```python
from build123d import *

# Parameters (mm, degrees)
F0_R     = 21.6611468636
F1_DEPTH = 12
F5_DEPTH = 15
F8_DEPTH = 32.9
F9_DEPTH = 5


with BuildPart() as f1:
    # F0 (on Top) → F1 (new body)
    with BuildSketch(Plane.XY):
        Polygon((-20.2222224325, 30.916666612), (-27.0277783275, 30.916666612), (-27.0277783275, 0), (-27.0277783275, -30.916666612), (-20.2222224325, -30.916666612), (-10.3055555373, -25.6666671485), (0, -25.6666671485), (10.3055555373, -25.6666671485), (20.2222224325, -30.916666612), (27.0277783275, -30.916666612), (27.0277783275, 0), (27.0277783275, 30.916666612), (20.2222224325, 30.916666612), (10.3055555373, 25.6666671485), (0, 25.6666671485), (-10.3055555373, 25.6666671485), align=None)
        Circle(F0_R, mode=Mode.SUBTRACT)
        Circle(F0_R)
    extrude(amount=-F1_DEPTH)

    # F4 (on plane+point) → F5 (join)
    with BuildSketch(Plane(origin=(-27.0277783275, 0, 0), x_dir=(0, -1, 0), z_dir=(-1, 0, 0))):
        with BuildLine():
            ThreePointArc((-37.3333357275, 1.750000054), (-45.7916693995, -6.708333618), (-37.3333357275, -15.16666729))
            Line((-37.3333357275, -15.16666729), (37.138890475, -15.16666729))
            ThreePointArc((37.138890475, -15.16666729), (45.5972241471, -6.708333618), (37.138890475, 1.750000054))
            Line((37.138890475, 1.750000054), (-37.3333357275, 1.750000054))
        make_face()
    extrude(amount=F5_DEPTH)

    # F6: F1 across plane


with BuildPart() as f1_1:
    add(f1.part)
    add(f1.part.mirror(Plane.YZ))

    # F7 (on Front) → F8 (cut, symmetric)
    with BuildSketch(Plane.XZ):
        Polygon((11.4722223952, -5.0555560738), (0, -5.0555560738), (-11.4722223952, -5.0555560738), (-24.1111125797, -13.6111117899), (0, -13.6111117899), (24.1111125797, -13.6111117899), align=None)
    extrude(amount=F8_DEPTH, both=True, mode=Mode.SUBTRACT)

    # F0 (on Top) → F9 (join)
    with BuildSketch(Plane.XY):
        Circle(F0_R)
    extrude(amount=F9_DEPTH)


solid = f1_1.part
```
Work out the finished part from the listing and answer in its coordinate system (mm). A direction names the side the tool comes from. Coordinates: 2 decimals unless noted, no trailing zeros. Order: outer loops, then holes, each group sorted by start corner. A loop starts at its lowest first (then second) coordinate and runs counter-clockwise, first axis right, second up. Notation, with made-up numbers: (79, -35.75) - (125, -35.75) arc R35 ccw to (125, -2.75) - close; hole circle Ø4 at (-25, -23.75). An arc over 180 degrees is marked (long way). Answer as a JSON object with one key per item and string values.
1. Consider line 1 (X direction, y = 42, z = -9); line 2 (Z direction, x = -36.5, y = -20); line 3 (X direction, y = -26.5, z = -7). Determine where each line is inside the solid, lowest interval first.
Output values:
{"line 1": "x = -42.03 to -27.03, 27.03 to 42.03", "line 2": "z = -15.17 to 1.75", "line 3": "x = -42.03 to -14.34, 14.34 to 42.03"}
2. Each of these flat-tipped pins is pushed along its axis until it touches: P1, Ø2, axis at x = -22.5, z = -5.5, coming from the +Y side; P2, Ø4, axis at x = 0, z = -1.5, coming from the +Y side; P3, Ø5, axis at x = 25, y = -6.5, coming from the -Z side; P4, Ø7, axis at x = 4.5, y = 4, coming from the -Z side. Where does it stop, or does it pass through?
Output values:
{"P1": "stops at y = 30.92", "P2": "stops at y = 25.67", "P3": "stops at z = -15.17", "P4": "stops at z = -5.06"}
3. Find section B-B on y = -34. Determine the outline of the cut face in (x, z), plus the area to 4 significant figures.
Output values:
{"outline": "(-42.03, -15.17) - (-27.03, -15.17) - (-27.03, 1.75) - (-42.03, 1.75) - close; (27.03, -15.17) - (42.03, -15.17) - (42.03, 1.75) - (27.03, 1.75) - close", "area": "507.5 mm²"}
4. Find section D-D on z = -3. Determine the outline of the cut face in (x, y), plus the area to 3 significant figures.
Output values:
{"outline": "(-42.03, -44.74) - (-27.03, -44.74) - (-27.03, -30.92) - (-20.22, -30.92) - (-10.31, -25.67) - (10.31, -25.67) - (20.22, -30.92) - (27.03, -30.92) - (27.03, -44.74) - (42.03, -44.74) - (42.03, 44.94) - (27.03, 44.94) - (27.03, 30.92) - (20.22, 30.92) - (10.31, 25.67) - (-10.31, 25.67) - (-20.22, 30.92) - (-27.03, 30.92) - (-27.03, 44.94) - (-42.03, 44.94) - close", "area": "5,710 mm²"}
5. Find section A-A on y = -24. Determine the outline of the cut face in (x, z), plus the area to 3 significant figures.
Output values:
{"outline": "(-42.03, -15.17) - (-27.03, -15.17) - (-27.03, -12) - (-21.73, -12) - (-11.47, -5.06) - (11.47, -5.06) - (21.73, -12) - (27.03, -12) - (27.03, -15.17) - (42.03, -15.17) - (42.03, 1.75) - (27.03, 1.75) - (27.03, 0) - (-27.03, 0) - (-27.03, 1.75) - (-42.03, 1.75) - close", "area": "926 mm²"}
6. A tool of negligible diameter and unlimited length cuts with its end or side. For faces 4 (the face through (24, 30.917, -6)), 5 (the face through (-34, 0, 1.75)), 6 (the face through (16.673, -0.433, -8.576)), 7 (the face through (-6, 21, 0)), 8 (the face through (0, -25.667, -2)), from which of +Z, -Z, +X, -X, +Y, -Y can it reach the whole face along a straight path? Write none if from no direction.
Output values:
{"face 4": "+Z, -Z, +Y", "face 5": "+Z, -X, +Y, -Y", "face 6": "-Z, +Y, -Y", "face 7": "+Z", "face 8": "+Z, -Z, -Y"}
7. Find section C-C on x = 0. Determine the outline of the cut face in (y, z).
Output values:
{"outline": "(-25.67, -5.06) - (25.67, -5.06) - (25.67, 0) - (21.66, 0) - (21.66, 5) - (-21.66, 5) - (-21.66, 0) - (-25.67, 0) - close"}
8. The mould has two halves that part along X. Classify faces 1 (the face through (34, 0, 1.75)), 2 (the face through (-42.028, 1, -7)), 3 (the face through (-16.53, -0.43, -8.48)): +X half, -X half, draft (parallel to the pull), parting line (faces both ways), or undercut.
Output values:
{"face 1": "draft", "face 2": "-X half", "face 3": "undercut"}
